```python
from build123d import *

# Parameters (mm, degrees)
SKETCH_1_W            = 60
SKETCH_1_H            = 60
EXTRUDE_1_DEPTH       = 2
EXTRUDE_2_DEPTH       = 4
MIRROR_2_COPY_1_DEPTH = 4
EXTRUDE_3_DEPTH       = 4
MIRROR_4_COPY_1_DEPTH = 4
FILLET_1_R            = 2


with BuildPart() as part:
    # 草图1 → 凸台-拉伸1 (new body)
    with BuildSketch(Plane(origin=(0, 0, 0), x_dir=(1, 0, 0), z_dir=(0, 1, 0))):
        Rectangle(SKETCH_1_W, SKETCH_1_H)
    extrude(amount=EXTRUDE_1_DEPTH)

    # 草图2 → 凸台-拉伸2 (add)
    with BuildSketch(Plane.XZ):
        with BuildLine():
            Line((-28.5, 13), (-28.5, 17))
            ThreePointArc((-28.5, 17), (-26.5, 15), (-28.5, 13))
        make_face()
    extrude_2 = extrude(amount=EXTRUDE_2_DEPTH)

    # 镜向1: 凸台-拉伸2 across plane
    add(extrude_2.mirror(Plane.XY))

    # 镜向2: 凸台-拉伸2 across plane
    add(extrude_2.mirror(Plane(origin=(0, 0, 0), x_dir=(0, 0, 1), z_dir=(1, 0, 0))))

    # 镜向2 copy 1 sketch → 镜向2 copy 1 (add)
    with BuildSketch(Plane(origin=(0, 0, 0), x_dir=(-1, 0, 0), z_dir=(0, -1, 0))):
        with BuildLine():
            Line((-28.5, 13), (-28.5, 17))
            ThreePointArc((-28.5, 17), (-26.5, 15), (-28.5, 13))
        make_face()
    extrude(amount=MIRROR_2_COPY_1_DEPTH)

    # 草图3 → 凸台-拉伸3 (add)
    with BuildSketch(Plane.XZ):
        with BuildLine():
            Line((-13, 28.5), (-17, 28.5))
            ThreePointArc((-17, 28.5), (-15, 26.5), (-13, 28.5))
        make_face()
    extrude_3 = extrude(amount=EXTRUDE_3_DEPTH)

    # 镜向3: 凸台-拉伸3 across plane
    add(extrude_3.mirror(Plane(origin=(0, 0, 0), x_dir=(0, 0, 1), z_dir=(1, 0, 0))))

    # 镜向4: 凸台-拉伸3 across plane
    add(extrude_3.mirror(Plane.XY))

    # 镜向4 copy 1 sketch → 镜向4 copy 1 (add)
    with BuildSketch(Plane(origin=(0, 0, 0), x_dir=(-1, 0, 0), z_dir=(0, -1, 0))):
        with BuildLine():
            Line((-13, 28.5), (-17, 28.5))
            ThreePointArc((-17, 28.5), (-15, 26.5), (-13, 28.5))
        make_face()
    extrude(amount=MIRROR_4_COPY_1_DEPTH)

    # 圆角1
    fillet_1_edges = [part.edges().sort_by_distance(p)[0] for p in [
        (0, 2, 30),
        (30, 2, 0),
        (0, 2, -30),
        (-30, 2, 0),
        (30, 1, -30),
        (30, 1, 30),
        (-30, 1, 30),
        (-30, 1, -30),
    ]]
    fillet(fillet_1_edges, radius=FILLET_1_R - 0.0001)  # a hair under: the kernel refuses the full size


solid = part.part
```
Here's how the part is built. I have some questions about the finished solid (model axes, mm). A direction names the side the tool comes from. Give positions to 0.01 mm unless a question says otherwise; leave off trailing zeros. Loops run counter-clockwise (first coordinate to the right, second up) from the corner with the lowest first, then second, coordinate; pieces in that order, holes last. Notation, with made-up numbers: (-32.75, 39.25) -> (24.25, 39.25) arc R35 cw to (24.25, 78.25) -> close; hole circle Ø10 at (43.25, 26). An arc over 180 degrees is marked (long way). Use one line per item in the form item = value. Start each with the question number.
1) For P1, Ø2, axis at x = -15.5, y = -2, coming from the -Z side; P2, Ø1, axis at x = 16, z = 3, coming from the -Y side; P3, Ø3, axis at y = -2, z = 16, coming from the +X side, each with a flat end and sliding along its axis, tell me the tip position at first contact or that it passes through.
2) Please list where these lines run through material, in increasing order: line 1 along Y through (x, z) = (5, -9); line 2 along X through (y, z) = (-2, 28); line 3 along X through (y, z) = (-2.05, 15.5).
3) Thinking about a two-plate mould opening in X: for faces 1 (the face through (15, -2, 26.5)), 2 (the face through (28, -4, 15)), 3 (the face through (28.5, -2, 15)), which applies, +X half, -X half, draft (parallel to the pull), parting line (faces both ways), or undercut?
4) Which directions (+Z, -Z, +X, -X, +Y, -Y) give clear straight access to the entire face, cutting with the end or side of a thin tool? Please do faces 4 (the face through (15, -2, -26.5)), 5 (the face through (15, -2, -28.5)), 6 (the face through (-15, -2, 28.5)).
5) Imagine slicing it at A-A (y = -1.65). Please give me the cut outline in (x, z).
Check values:
q1.P1 = -28.5
q1.P2 = 0
q1.P3 = 28.5
q2.line_1 = 0 to 2
q2.line_2 = -16.94 to -13.06, 13.06 to 16.94
q2.line_3 = -28.5 to -26.56, 26.56 to 28.5
q3.face_1 = undercut
q3.face_2 = draft
q3.face_3 = +X half
q4.face_4 = -Y
q4.face_5 = -Z, +X, -X, -Y
q4.face_6 = +Z, +X, -X, -Y
q5.outline = (-28.5, -17) arc R2 ccw to (-28.5, -13) -> close; (-28.5, 13) arc R2 ccw to (-28.5, 17) -> close; (-17, -28.5) -> (-13, -28.5) arc R2 ccw to start; (-17, 28.5) arc R2 ccw to (-13, 28.5) -> close; (13, -28.5) -> (17, -28.5) arc R2 ccw to start; (13, 28.5) arc R2 ccw to (17, 28.5) -> close; (28.5, -17) -> (28.5, -13) arc R2 ccw to start; (28.5, 13) -> (28.5, 17) arc R2 ccw to start
